```python
from build123d import *

# Parameters (mm, degrees)
BOSS_EXTRUDE1_DEPTH = 3.5
FILLET1_R           = 1


with BuildPart() as part:
    # Sketch1 → Boss-Extrude1 (new body)
    with BuildSketch(Plane.XY):
        with BuildLine():
            Line((-6, -5), (-4, -5))
            Line((-4, -5), (-4, -3))
            ThreePointArc((-4, -3), (0, 1), (4, -3))
            Line((4, -3), (4, -5))
            Line((4, -5), (6, -5))
            ThreePointArc((6, -5), (7.414213562, -4.414213562), (8, -3))
            Line((8, -3), (8, 3))
            ThreePointArc((8, 3), (7.414213562, 4.414213562), (6, 5))
            Line((6, 5), (-6, 5))
            ThreePointArc((-6, 5), (-7.414213562, 4.414213562), (-8, 3))
            Line((-8, 3), (-8, -3))
            ThreePointArc((-8, -3), (-7.414213562, -4.414213562), (-6, -5))
        make_face()
    extrude(amount=BOSS_EXTRUDE1_DEPTH)

    # Fillet1
    fillet1_edges = [part.edges().sort_by_distance(p)[0] for p in [
        (-4, -5, 1.75),
        (4, -5, 1.75),
    ]]
    fillet(fillet1_edges, radius=FILLET1_R)


solid = part.part
```
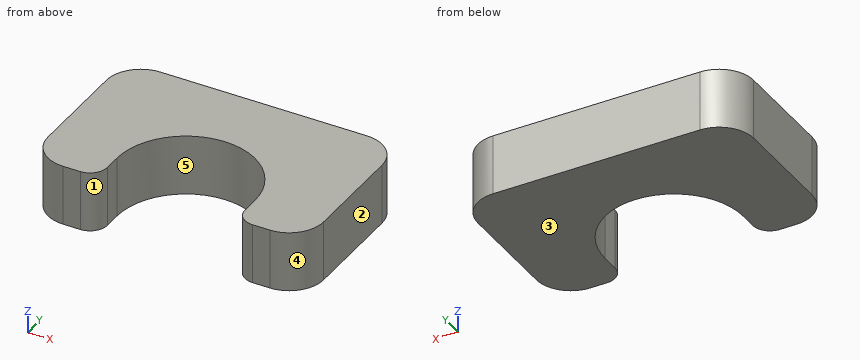
Geometry: final body of the model. Coordinates: model frame, mm. Face numbers are marked on the shaded views. A direction names the side the tool comes from. Give positions to 0.01 mm unless a question says otherwise; leave off trailing zeros. Loops run counter-clockwise (first coordinate to the right, second up) from the corner with the lowest first, then second, coordinate; pieces in that order, holes last. Notation, with made-up numbers: (35, -13.5) -> (89, -13.5) arc R31 cw to (89, 17.5) -> close; hole circle Ø9 at (-40, 49). An arc over 180 degrees is marked (long way). Use CSV: the item, a comma, the result in double quotes.
(1) Access query for the marked faces 1 and 2. Directions: +Z, -Z, +X, -X, +Y, -Y. A direction counts if a zero-diameter tool reaches every point of the face in a straight line with its end or side. Return the directions, or none.
From the geometry:
face 1,"+Z, -Z, -Y"
face 2,"+Z, -Z, +X, +Y, -Y"
(2) Cut plane B-B (y = -3.25). Output: boundary loops of the cut face in (x, z), plus the area to 3 significant figures.
From the geometry:
outline,"(-7.98, 0) -> (-4, 0) -> (-4, 3.5) -> (-7.98, 3.5) -> close; (4, 0) -> (7.98, 0) -> (7.98, 3.5) -> (4, 3.5) -> close"
area,"27.9 mm^2"
(3) Cut plane C-C (x = 0). Output: boundary loops of the cut face in (y, z), plus the area to 3 significant figures.
From the geometry:
outline,"(1, 0) -> (5, 0) -> (5, 3.5) -> (1, 3.5) -> close"
area,"14.0 mm^2"
(4) Cut plane D-D (y = 0.25). Output: boundary loops of the cut face in (x, z), plus the area to 3 significant figures.
From the geometry:
outline,"(-8, 0) -> (-2.33, 0) -> (-2.33, 3.5) -> (-8, 3.5) -> close; (2.33, 0) -> (8, 0) -> (8, 3.5) -> (2.33, 3.5) -> close"
area,"39.7 mm^2"
(5) Cut plane A-A (z = 1.9). Output: boundary loops of the cut face in (x, y).
From the geometry:
outline,"(-8, -3) arc R2 ccw to (-6, -5) -> (-5, -5) arc R1 ccw to (-4, -4) -> (-4, -3) arc R4 cw to (4, -3) -> (4, -4) arc R1 ccw to (5, -5) -> (6, -5) arc R2 ccw to (8, -3) -> (8, 3) arc R2 ccw to (6, 5) -> (-6, 5) arc R2 ccw to (-8, 3) -> close"
(6) Pull-direction query (X, two-part tool) for the marked faces 3, 4 and 5; classes: released by +X, released by -X, zero draft, split by the parting line, or undercut.
From the geometry:
face 3,"zero draft"
face 4,"released by +X"
face 5,"undercut"
(7) Ray query, line 1 along X through (y, z) = (-3, 1.2); line 2 along X through (y, z) = (0, 1.25); line 3 along X through (y, z) = (4, 2.65). Return the intervals inside material, ascending. Write a range as [from, to].
From the geometry:
line 1,"[-8, -4], [4, 8]"
line 2,"[-8, -2.65], [2.65, 8]"
line 3,"[-7.73, 7.73]"
